For this review, take the finished solid that the model builds, in its own axes (mm). Face numbers are marked on the shaded views. Coordinates: 2 decimals unless noted, no trailing zeros. Write each loop counter-clockwise with the first axis right and the second up, starting at its lowest first coordinate (ties: lowest second). Pieces come first, ordered by that corner, then holes.
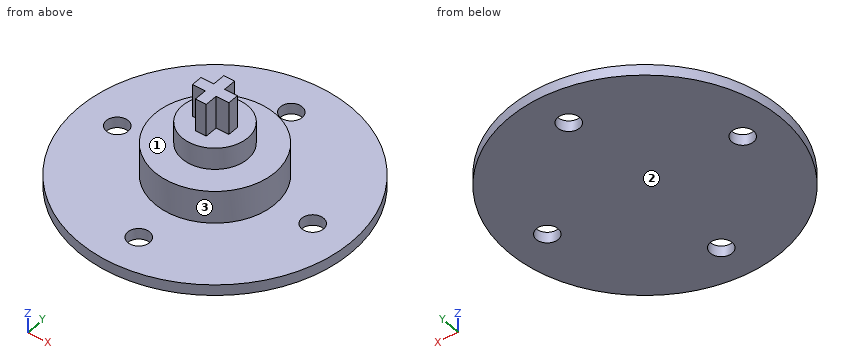
```python
from build123d import *

# Parameters (mm, degrees)
F0_R     = 12.5
F0_R_2   = 1
F1_DEPTH = 1
F2_R     = 5.5
F3_DEPTH = 3
F4_R     = 3
F5_DEPTH = 2
F6_W     = 1
F6_H     = 1.1770509831
F6_H_2   = 1
F6_W_2   = 1.1770509831
F7_DEPTH = 3


with BuildPart() as f1:
    # F0 (on Top) → F1 (new body)
    with BuildSketch(Plane.XY):
        Circle(F0_R)
        with Locations((0, -9)):
            Circle(F0_R_2, mode=Mode.SUBTRACT)
        with Locations((-9, 0)):
            Circle(F0_R_2, mode=Mode.SUBTRACT)
        with Locations((9, 0)):
            Circle(F0_R_2, mode=Mode.SUBTRACT)
        with Locations((0, 9)):
            Circle(F0_R_2, mode=Mode.SUBTRACT)
    extrude(amount=F1_DEPTH)

    # F2 (on face) → F3 (join)
    with BuildSketch(Plane.XY.offset(1)):
        Circle(F2_R)
    extrude(amount=F3_DEPTH)

    # F4 (on face) → F5 (join)
    with BuildSketch(Plane.XY.offset(4)):
        Circle(F4_R)
    extrude(amount=F5_DEPTH)

    # F6 (on face) → F7 (join)
    with BuildSketch(Plane.XY.offset(6)):
        with Locations((0, 1.0885254916)):
            Rectangle(F6_W, F6_H)
        Rectangle(F6_W, F6_H_2)
        with Locations((-1.0885254916, 0)):
            Rectangle(F6_W_2, F6_H_2)
        with Locations((1.0885254916, 0)):
            Rectangle(F6_W_2, F6_H_2)
        with Locations((0, -1.0885254916)):
            Rectangle(F6_W, F6_H)
    extrude(amount=F7_DEPTH)


solid = f1.part
```
Q1. Clearance check with flat-ended pins moving along their axes: pin 1 Ø1.3 at (y, z) = (1, 7) entering from +X; pin 2 Ø3 at (y, z) = (9.5, 1) entering from +X; pin 3 Ø1.3 at (x, z) = (-1, 8) entering from +Y. State where each tip first meets the part, or that it passes through.
Ans:
pin 1: stops at x = 1.68
pin 2: stops at x = 9.6
pin 3: stops at y = 1.68
Q2. Add section A-A (y = 0). State the section outline as (x, z) points, then the cut area to 3 significant figures.
Ans:
outline: (-12.5, 0) - (-10, 0) - (-10, 1) - (-12.5, 1) - close; (-8, 0) - (8, 0) - (8, 1) - (5.5, 1) - (5.5, 4) - (3, 4) - (3, 6) - (1.68, 6) - (1.68, 9) - (-1.68, 9) - (-1.68, 6) - (-3, 6) - (-3, 4) - (-5.5, 4) - (-5.5, 1) - (-8, 1) - close; (10, 0) - (12.5, 0) - (12.5, 1) - (10, 1) - close
area: 76.1 mm2
Q3. Draft analysis for pull direction Z (two halves, no side actions). For the marked faces 1, 2 and 3, state which applies: +Z half, -Z half, draft (parallel to the pull), parting line (faces both ways), or undercut.
Ans:
face 1: +Z half
face 2: -Z half
face 3: draft
Q4. Add section D-D (x = 9). State the section outline as (y, z) points, then the cut area to 3 significant figures.
Ans:
outline: (-8.67, 0) - (-1, 0) - (-1, 1) - (-8.67, 1) - close; (1, 0) - (8.67, 0) - (8.67, 1) - (1, 1) - close
area: 15.3 mm2
Q5. Add section B-B (z = 6.75). State the section outline as (x, y) points.
Ans:
outline: (-1.68, -0.5) - (-0.5, -0.5) - (-0.5, -1.68) - (0.5, -1.68) - (0.5, -0.5) - (1.68, -0.5) - (1.68, 0.5) - (0.5, 0.5) - (0.5, 1.68) - (-0.5, 1.68) - (-0.5, 0.5) - (-1.68, 0.5) - close
Q6. For probe 1 along Y at (x, z) = (0, 0.65); probe 2 along Z at (x, y) = (-1, 4); probe 3 along Z at (x, y) = (-11, -2.25), list the stretches that pass through material, from the lowest coordinate up.
Ans:
probe 1: y = -12.5 to -10, -8 to 8, 10 to 12.5
probe 2: z = 0 to 4
probe 3: z = 0 to 1
